from build123d import *

# Parameters (mm, degrees)
SKETCH1_W           = 12
SKETCH1_H           = 20
SKETCH1_W_2         = 10
SKETCH1_H_2         = 18
BOSS_EXTRUDE1_DEPTH = 450
CUT_EXTRUDE1_REACH  = 452.271
SKETCH2_R           = 1.5
SKETCH3_R           = 1.5
CUT_EXTRUDE2_DEPTH  = 451.484183962


with BuildPart() as part:
    # Sketch1 → Boss-Extrude1 (new body)
    with BuildSketch(Plane.XY):
        Rectangle(SKETCH1_W, SKETCH1_H)
        Rectangle(SKETCH1_W_2, SKETCH1_H_2, mode=Mode.SUBTRACT)
    extrude(amount=BOSS_EXTRUDE1_DEPTH)

    # Sketch2 → Cut-Extrude1 (cut, up to next)
    with BuildSketch(Plane(origin=(6, 0, 0), x_dir=(0, 0, -1), z_dir=(1, 0, 0)), mode=Mode.PRIVATE) as cut_extrude1_sk1:
        with Locations((-168, 0)):
            Circle(SKETCH2_R)
    cut_extrude1_tool1 = extrude(cut_extrude1_sk1.sketch, amount=-CUT_EXTRUDE1_REACH, mode=Mode.PRIVATE) & part.part
    # Sketch2 → Cut-Extrude1 (cut, up to next)
    with BuildSketch(Plane(origin=(6, 0, 0), x_dir=(0, 0, -1), z_dir=(1, 0, 0)), mode=Mode.PRIVATE) as cut_extrude1_sk2:
        with Locations((-150, 0)):
            Circle(SKETCH2_R)
    cut_extrude1_tool2 = extrude(cut_extrude1_sk2.sketch, amount=-CUT_EXTRUDE1_REACH, mode=Mode.PRIVATE) & part.part
    # Sketch2 → Cut-Extrude1 (cut, up to next)
    with BuildSketch(Plane(origin=(6, 0, 0), x_dir=(0, 0, -1), z_dir=(1, 0, 0)), mode=Mode.PRIVATE) as cut_extrude1_sk3:
        with Locations((-132, 0)):
            Circle(SKETCH2_R)
    cut_extrude1_tool3 = extrude(cut_extrude1_sk3.sketch, amount=-CUT_EXTRUDE1_REACH, mode=Mode.PRIVATE) & part.part
    add(cut_extrude1_tool1.solids().sort_by_distance((6, 0, 168))[0], mode=Mode.SUBTRACT)
    add(cut_extrude1_tool2.solids().sort_by_distance((6, 0, 150))[0], mode=Mode.SUBTRACT)
    add(cut_extrude1_tool3.solids().sort_by_distance((6, 0, 132))[0], mode=Mode.SUBTRACT)

    # Sketch3 → Cut-Extrude2 (cut, through all)
    with BuildSketch(Plane(origin=(0, 10, 0), x_dir=(1, 0, 0), z_dir=(0, 1, 0))):
        with Locations(Location((0, -444, 0), (0, 0, 270))):
            Circle(SKETCH3_R)
        with Locations(Location((0, -420, 0), (0, 0, 270))):
            Circle(SKETCH3_R)
        with Locations(Location((0, -24, 0), (0, 0, 270))):
            Circle(SKETCH3_R)
        with Locations(Location((0, -72, 0), (0, 0, 270))):
            Circle(SKETCH3_R)
    extrude(amount=-CUT_EXTRUDE2_DEPTH, mode=Mode.SUBTRACT)


solid = part.part
Part model, mm, in its own coordinate system. A direction names the side the tool comes from. Give positions to 0.01 mm unless a question says otherwise; leave off trailing zeros. Order: outer loops, then holes, each group sorted by start corner. A loop starts at its lowest first (then second) coordinate and runs counter-clockwise, first axis right, second up. Notation, with made-up numbers: (46, -28.5) -> (55, -28.5) arc R11 ccw to (55, -12.5) -> close; hole circle Ø9 at (14, 29). An arc over 180 degrees is marked (long way). Use one line per item in the form item = value.
(1) Flat gauge pins, fed straight in: P1, Ø2.5, axis at x = 0, z = 420, coming from the +Y side; P2, Ø2.5, axis at y = 0, z = 132, coming from the +X side. Where does each tip first touch, or does it go through?
Solution:
P1 = through
P2 = -5
(2) Pull direction Y, two halves, no side cores. Call faces 3 (the face through (0, -10, 222)), 4 (the face through (5, 0, 222)), 5 (the face through (-5.4, 0.8, 0)): +Y half, -Y half, draft (parallel to the pull), parting line (faces both ways), or undercut.
Solution:
face_3 = -Y half
face_4 = undercut
face_5 = draft
(3) Saw through at A-A (z = 225.5). Write the cut outline in (x, y), then the cut area to 3 significant figures.
Solution:
outline = (-6, -10) -> (6, -10) -> (6, 10) -> (-6, 10) -> close; hole (-5, -9) -> (5, -9) -> (5, 9) -> (-5, 9) -> close
area = 60.0 mm²
(4) Tool access for faces 1 (the face through (-6, 0, 222)), 2 (the face through (-5, 0, 222)): list every direction of +Z, -Z, +X, -X, +Y, -Y with a clear straight run to the whole face (end or side of a thin tool).
Solution:
face_1 = +Z, -Z, -X, +Y, -Y
face_2 = +Z, -Z
(5) Drill centre lines: line 1 (X direction, y = 9.2, z = 420); line 2 (Y direction, x = -2.25, z = 102); line 3 (Y direction, x = 5.45, z = 168). Where is each one in solid material? Low to high. Write a range as from..to.
Solution:
line_1 = -6..-1.5, 1.5..6
line_2 = -10..-9, 9..10
line_3 = -10..-1.5, 1.5..10
